CAD build for the part. Positions are in the model's coordinates, mm. A direction names the side the tool comes from. Round coordinates to 2 decimals unless told otherwise and drop trailing zeros. Loops run counter-clockwise (first coordinate to the right, second up) from the corner with the lowest first, then second, coordinate; pieces in that order, holes last.
```python
from build123d import *

# Parameters (mm, degrees)
CUT_EXTRUDE3_DEPTH           = 60
CUT_EXTRUDE5_DEPTH           = 2
CUT_EXTRUDE5_DEPTH_BACK      = 30
SKETCH9_R                    = 38
SKETCH9_R_2                  = 23
SKETCH19_W                   = 12
SKETCH19_H                   = 36.5
CUT_REVOLVE2_ANGLE           = 65
CUT_REVOLVE2_OTHER_WAY_ANGLE = 65
SKETCH21_W                   = 3.25
SKETCH21_H                   = 4
BOSS_EXTRUDE3_DEPTH          = 1.35
CIRPATTERN1_COUNT            = 5
CUT_EXTRUDE9_START           = -5
CUT_EXTRUDE9_DEPTH           = 5
SKETCH23_R                   = 10.5
CUT_EXTRUDE10_DEPTH          = 10
SKETCH24_W                   = 17
SKETCH24_H                   = 12
BOSS_EXTRUDE4_DEPTH          = 8
SKETCH26_W                   = 12
SKETCH26_H                   = 8
CUT_EXTRUDE11_DEPTH          = 10
SKETCH27_W                   = 4
SKETCH27_H                   = 5
CUT_EXTRUDE12_DEPTH          = 5
CUT_EXTRUDE14_DEPTH          = 2
CUT_EXTRUDE14_DEPTH_BACK     = 30
SKETCH29_R                   = 1
CUT_EXTRUDE15_DEPTH          = 15
FILLET1_R                    = 6
FILLET2_R                    = 8
INTERSECT2_DEPTH             = 58.427876097


# Read off the part's stored shape, not the designer's step: Cut-Extrude9, Intersect2
with BuildPart() as part:
    # Sketch1 → Revolve1 (revolve)
    with BuildSketch(Plane.XY, mode=Mode.PRIVATE) as revolve1_sk:
        with BuildLine():
            Line((0, 63.427876097), (32, 63.427876097))
            ThreePointArc((32, 63.427876097), (37.656854249, 61.084730346), (40, 55.427876097))
            Line((40, 55.427876097), (40, 28.846818009))
            ThreePointArc((40, 28.846818009), (38.792081772, 24.082439968), (35.460140376, 20.469057744))
            Line((35.460140376, 20.469057744), (28.539859624, 15.958818353))
            ThreePointArc((28.539859624, 15.958818353), (25.207918228, 12.345436129), (24, 7.581058088))
            Line((24, 7.581058088), (24, 3.25))
            Line((24, 3.25), (24.35, 3))
            Line((24.35, 3), (24.35, 0))
            Line((24.35, 0), (22.5, 0))
            Line((22.5, 0), (22.5, 12.5))
            ThreePointArc((22.5, 12.5), (22.353553391, 12.853553391), (22, 13))
            Line((22, 13), (0, 13))
            Line((0, 13), (0, 63.427876097))
        make_face()
    revolve(revolve1_sk.sketch.rotate(Axis((0, 0, 0), (0, 1, 0)), 90), axis=Axis((0, 0, 0), (0, 1, 0)))

    # Sketch11 → Cut-Extrude3 (cut)
    with BuildSketch(Plane(origin=(0, 13, 0), x_dir=(-1, 0, 0), z_dir=(0, -1, 0))):
        with BuildLine():
            Line((-21, 0), (21, 0))
            ThreePointArc((21, 0), (0, 21), (-21, 0))
        make_face()
    extrude(amount=-CUT_EXTRUDE3_DEPTH, mode=Mode.SUBTRACT)

    # Sketch9 → Cut-Extrude5 (cut, two sides: drawn at the far end of the back side and taken through both)
    with BuildSketch(Plane(origin=(0, 55.427876097, 0), x_dir=(1, 0, 0), z_dir=(0, 1, 0)).offset(-CUT_EXTRUDE5_DEPTH_BACK)):
        with Locations(Location((0, 0, 0), (0, 0, 270))):
            Circle(SKETCH9_R)
        with Locations(Location((0, 0, 0), (0, 0, 270))):
            Circle(SKETCH9_R_2, mode=Mode.SUBTRACT)
    extrude(amount=CUT_EXTRUDE5_DEPTH + CUT_EXTRUDE5_DEPTH_BACK, mode=Mode.SUBTRACT)

    # Sketch19 → Cut-Revolve2 (revolve, cut)
    with BuildSketch(Plane(origin=(0, 0, 0), x_dir=(0, 0, -1), z_dir=(1, 0, 0))):
        with Locations((-41.064715832, 37.177876097)):
            Rectangle(SKETCH19_W, SKETCH19_H)
    revolve(axis=Axis((0, 0, 0), (0, 1, 0)), revolution_arc=CUT_REVOLVE2_ANGLE, mode=Mode.SUBTRACT)

    # Sketch19 → Cut-Revolve2 other way (revolve, cut)
    with BuildSketch(Plane(origin=(0, 0, 0), x_dir=(0, 0, -1), z_dir=(1, 0, 0))):
        with Locations((-41.064715832, 37.177876097)):
            Rectangle(SKETCH19_W, SKETCH19_H)
    revolve(axis=Axis((0, 0, 0), (0, -1, 0)), revolution_arc=CUT_REVOLVE2_OTHER_WAY_ANGLE, mode=Mode.SUBTRACT)

    # Sketch21 → Boss-Extrude3 (add)
    with BuildSketch(Plane(origin=(0, 0, 22.5), x_dir=(-1, 0, 0), z_dir=(0, 0, -1))):
        with Locations((0, 2)):
            Rectangle(SKETCH21_W, SKETCH21_H)
    boss_extrude3 = extrude(amount=BOSS_EXTRUDE3_DEPTH)

    # CirPattern1: Boss-Extrude3 ×5 about axis
    cirpattern1_axis = Axis((0, 0, 0), (0, 1, 0))
    for i in range(1, CIRPATTERN1_COUNT):
        add(boss_extrude3.rotate(cirpattern1_axis, i * 360 / CIRPATTERN1_COUNT))

    # Cut-Extrude9 outline → Cut-Extrude9 (cut)
    with BuildSketch(Plane(origin=(0, 63.427876097, 0), x_dir=(1, 0, 0), z_dir=(0, 1, 0)).offset(CUT_EXTRUDE9_START)):
        with BuildLine():
            ThreePointArc((40, 0), (0, 40), (-40, 0))
            Line((-40, 0), (-21, 0))
            ThreePointArc((-21, 0), (0, 21), (21, 0))
            Line((21, 0), (40, 0))
        make_face()
    extrude(amount=CUT_EXTRUDE9_DEPTH, mode=Mode.SUBTRACT)

    # Sketch23 → Cut-Extrude10 (cut)
    with BuildSketch(Plane(origin=(0, 0, -40), x_dir=(-1, 0, 0), z_dir=(0, 0, -1))):
        with Locations((0, 42.137876097)):
            Circle(SKETCH23_R)
    extrude(amount=-CUT_EXTRUDE10_DEPTH, mode=Mode.SUBTRACT)

    # Sketch24 → Boss-Extrude4 (add)
    with BuildSketch(Plane(origin=(0, 58.427876097, 0), x_dir=(1, 0, 0), z_dir=(0, 1, 0))):
        with Locations((0, 30)):
            Rectangle(SKETCH24_W, SKETCH24_H)
    extrude(amount=-BOSS_EXTRUDE4_DEPTH)

    # Sketch26 → Cut-Extrude11 (cut)
    with BuildSketch(Plane(origin=(0, 58.427876097, 0), x_dir=(1, 0, 0), z_dir=(0, 1, 0))):
        with Locations((0, 30)):
            Rectangle(SKETCH26_W, SKETCH26_H)
    extrude(amount=-CUT_EXTRUDE11_DEPTH, mode=Mode.SUBTRACT)

    # Sketch27 → Cut-Extrude12 (cut)
    with BuildSketch(Plane(origin=(8.5, 0, 0), x_dir=(0, 0, -1), z_dir=(1, 0, 0))):
        with Locations((29.5, 53.927876097)):
            Rectangle(SKETCH27_W, SKETCH27_H)
    extrude(amount=-CUT_EXTRUDE12_DEPTH, mode=Mode.SUBTRACT)

    # Sketch28 → Cut-Extrude14 (cut, two sides: drawn at the far end of the back side and taken through both)
    with BuildSketch(Plane(origin=(0, 55.427876097, 0), x_dir=(1, 0, 0), z_dir=(0, 1, 0)).offset(-CUT_EXTRUDE14_DEPTH_BACK)):
        with BuildLine():
            Line((-22.912878475, -2), (22.912878475, -2))
            ThreePointArc((22.912878475, -2), (0, -23), (-22.912878475, -2))
        make_face()
    extrude(amount=CUT_EXTRUDE14_DEPTH + CUT_EXTRUDE14_DEPTH_BACK, mode=Mode.SUBTRACT)

    # Sketch29 → Cut-Extrude15 (cut)
    with BuildSketch(Plane(origin=(0, 0, 0), x_dir=(-1, 0, 0), z_dir=(0, 0, -1))):
        with Locations((-30.416198487, 60.927876097)):
            Circle(SKETCH29_R)
        with Locations((30.416198487, 60.927876097)):
            Circle(SKETCH29_R)
        with Locations((0, 60.927876097)):
            Circle(SKETCH29_R)
    extrude(amount=-CUT_EXTRUDE15_DEPTH, mode=Mode.SUBTRACT)

    # Fillet1
    fillet1_edges = [part.edges().sort_by_distance(p)[0] for p in [
        (21, 35.713938048, 0),
        (-21, 35.713938048, 0),
    ]]
    fillet(fillet1_edges, radius=FILLET1_R)

    # Fillet2
    fillet2_edges = [part.edges().sort_by_distance(p)[0] for p in [
        (-22.912878475, 41.427876097, 2),
        (22.912878475, 41.427876097, 2),
    ]]
    fillet(fillet2_edges, radius=FILLET2_R)

    # Intersect2 outline → Intersect2 (cut)
    with BuildSketch(Plane(origin=(0, 0, 0), x_dir=(1, 0, 0), z_dir=(0, 1, 0))):
        with BuildLine():
            Line((-37.508702776, -13.895942431), (-42, -15.355253362))
            Line((-42, -15.355253362), (-42, -41))
            Line((-42, -41), (42, -41))
            Line((42, -41), (42, -15.355253362))
            Line((42, -15.355253362), (37.508702776, -13.895942431))
            ThreePointArc((37.508702776, -13.895942431), (0, 40), (-37.508702776, -13.895942431))
        make_face()
        with BuildLine():
            ThreePointArc((19.246817919, 8.4), (18.767687244, 2.713664655), (13.747727085, 0))
            Line((13.747727085, 0), (-13.747727085, 0))
            ThreePointArc((-13.747727085, 0), (-18.767687244, 2.713664655), (-19.246817919, 8.4))
            ThreePointArc((-19.246817919, 8.4), (0, 21), (19.246817919, 8.4))
        make_face(mode=Mode.SUBTRACT)
    extrude(amount=INTERSECT2_DEPTH, mode=Mode.SUBTRACT)


solid = part.part
```
Item 1: Two-plate mould, pull along Y, no slides. Class faces 1 (the flat face through (1, 60, 0)), 2 (the flat face through (30, 61, 15)), 3 (the flat face through (0, 63.428, 12)): released by +Y, released by -Y, zero draft, split by the parting line, or undercut.
Answers follow:
face 1: zero draft
face 2: undercut
face 3: released by +Y
Item 2: Cut at A-A, the plane x = 0. Give the cut face in (y, z), plus the area to 3 significant figures.
Answers follow:
outline: (58.43, 0) - (59.93, 0) - (59.93, 15) - (61.93, 15) - (61.93, 0) - (63.43, 0) - (63.43, 32) arc R8 ccw to (58.43, 39.42) - close
area: 157 mm2
Item 3: Probe line 1 (X direction, y = 60.95, z = 10); line 2 (Y direction, x = 0, z = 4); line 3 (X direction, y = 61.55, z = 5). List the from-to ranges inside material, lowest first.
Answers follow:
line 1: x = -36.44 to -31.42, -29.42 to -1, 1 to 29.42, 31.42 to 36.44
line 2: y = 58.43 to 59.93, 61.93 to 63.43
line 3: x = -36.81 to -31.2, -29.63 to -0.78, 0.78 to 29.63, 31.2 to 36.81
Item 4: Cut at B-B, the plane z = 5. State how many separate pieces and enclosed holes the cut face has, plus the area to 3 significant figures.
Answers follow:
separate pieces: 1
enclosed holes: 3
area: 361 mm2
Item 5: Flat gauge pins, fed straight in: P1, Ø1.2, axis at x = -30.42, y = 60.93, coming from the +Z side; P2, Ø1.8, axis at x = 30.42, y = 60.93, coming from the -Z side; P3, Ø1, axis at x = 7, y = 59.5, coming from the +Z side. Where does each tip first touch, or does it go through?
Answers follow:
P1: stops at z = 23.62
P2: stops at z = 15
P3: stops at z = 38.54
Item 6: 3-axis set-ups, long thin cutter, end or side, ignore diameter. For faces 4 (the flat face through (-1, 58.428, 15)), 5 (the cylindrical face through (0.217, 59.952, 7.395)): which of +Z, -Z, +X, -X, +Y, -Y reach the whole face in a straight line?
Answers follow:
face 4: +Z, -Z, +X, -X, -Y
face 5: -Z
